Drawing for the job (mm, zero at the part's lowest x, y, z). A direction names the side the tool comes from. Give positions to 0.01 mm unless a question says otherwise; leave off trailing zeros. Order: outer loops, then holes, each group sorted by start corner. A loop starts at its lowest first (then second) coordinate and runs counter-clockwise, first axis right, second up. Notation, with made-up numbers: M -4.75,-22.75 L 50.25,-22.75 A30 cw 50.25,12.25 Z; hole C 35.25,38.5 d1. An arc over 180 degrees is marked long. Answer as a JSON object with one key per item and string values.
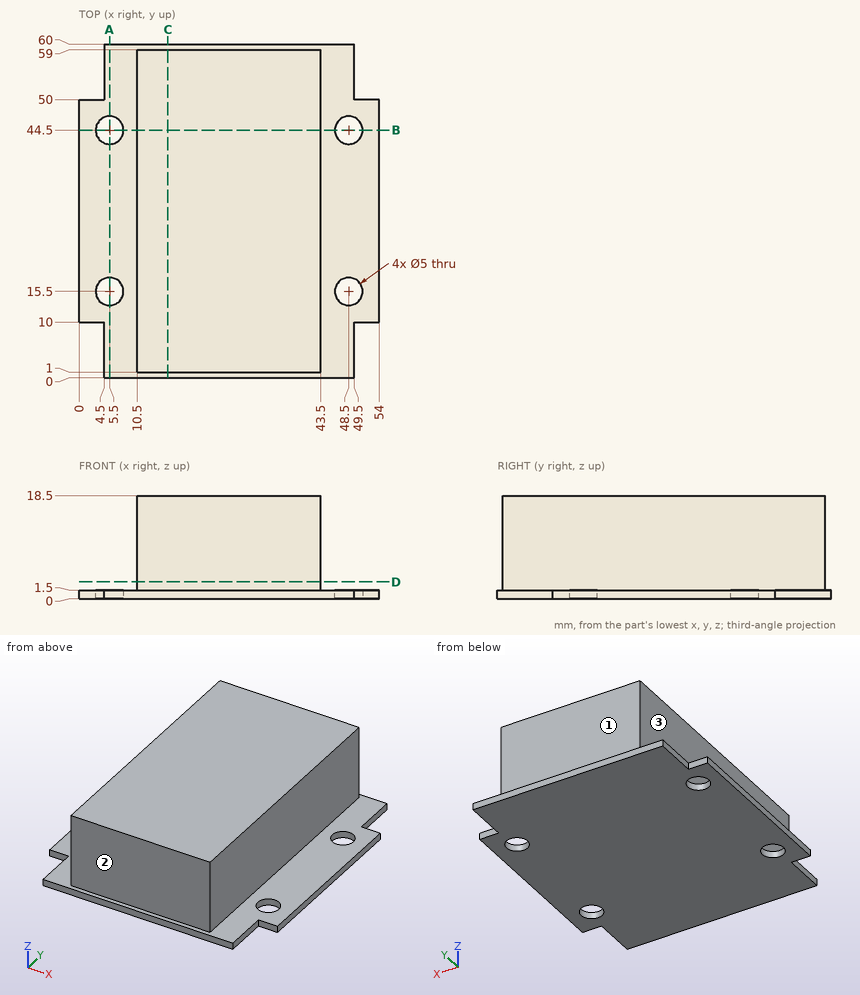
1. Probe line 1 along Y through (x, z) = (5.5, 0.9); line 2 along Z through (x, y) = (8, 30.5); line 3 along X through (y, z) = (19.5, 8). List the from-to ranges inside material, lowest first.
Worked answers:
{"line 1": "y = 0 to 13, 18 to 42, 47 to 60", "line 2": "z = 0 to 1.5", "line 3": "x = 10.5 to 43.5"}
2. Which spindle directions (+Z, -Z, +X, -X, +Y, -Y) get a long thin tool onto all of the face, cutting with end or side? Do the marked faces 1, 2 and 3. Say none if no direction does.
Worked answers:
{"face 1": "+Z, +X, -X, +Y", "face 2": "+Z, +X, -X, -Y", "face 3": "+Z, -X, +Y, -Y"}
3. Cut at A-A on x = 5.5. Give the cut face in (y, z).
Worked answers:
{"outline": "M 0,0 L 13,0 L 13,1.5 L 0,1.5 Z; M 18,0 L 42,0 L 42,1.5 L 18,1.5 Z; M 47,0 L 60,0 L 60,1.5 L 47,1.5 Z"}
4. Cut at D-D on z = 3. Give the cut face in (x, y).
Worked answers:
{"outline": "M 10.5,1 L 43.5,1 L 43.5,59 L 10.5,59 Z"}
5. Cut at B-B on y = 44.5. Give the cut face in (x, z).
Worked answers:
{"outline": "M 0,0 L 3,0 L 3,1.5 L 0,1.5 Z; M 8,0 L 46,0 L 46,1.5 L 43.5,1.5 L 43.5,18.5 L 10.5,18.5 L 10.5,1.5 L 8,1.5 Z; M 51,0 L 54,0 L 54,1.5 L 51,1.5 Z"}
6. Cut at C-C on x = 16. Give the cut face in (y, z), plus the area to 3 significant figures.
Worked answers:
{"outline": "M 0,0 L 60,0 L 60,1.5 L 59,1.5 L 59,18.5 L 1,18.5 L 1,1.5 L 0,1.5 Z", "area": "1,080 mm^2"}
7. Pin check, flat tips, straight feed: P1, Ø8, axis at x = 14.5, z = 8, coming from the +Y side; P2, Ø0.8, axis at y = 53.5, z = 0.5, coming from the +X side; P3, Ø4, axis at y = 46, z = 15.5, coming from the -X side. Stop position of each tip, or through.
Worked answers:
{"P1": "stops at y = 59", "P2": "stops at x = 49.5", "P3": "stops at x = 10.5"}
